Autodesk Inventor part; units mm, degrees
ref_plane "YZ Plane" through (0, 0, 0) normal (1, 0, 0) x (0, 1, 0)
ref_plane "XZ Plane" through (0, 0, 0) normal (0, 1, 0) x (-1, 0, 0)
ref_plane "XY Plane" through (0, 0, 0) normal (0, 0, 1) x (1, 0, 0)
sketch "Sketch1" plane through (0, 0, 0) normal (0, 0, 1) x (1, 0, 0)
  line L0 (0, 0) -> (120.65, 0)
  line L1 (120.65, 0) -> (120.65, 113.9317)
  line L2 (0, 113.9317) -> (0, 0)
  circle A0 centre (11.2141, 60.325) radius 1.9431
  circle A1 centre (60.325, 11.2141) radius 1.9431
  circle A2 centre (109.4359, 60.325) radius 1.9431
  circle A3 centre (60.325, 109.4359) radius 1.9431
  line L3 (60.071, 55.0418) -> (70.739, 55.0418)
  line L4 (70.739, 44.8818) -> (60.071, 44.8818)
  line L5 (60.071, 55.0418) -> (60.071, 44.8818)
  line L6 (70.739, 55.0418) -> (70.739, 44.8818)
  line L7 (60.325, 113.9317) -> (120.65, 113.9317)
  line L8 (60.325, 113.9317) -> (0, 113.9317)
  point P0 (60.325, 60.325)
  dimension "d10" = 3.8862
  dimension "d13" = 360
  dimension "d44" = 4.4958
extrude "Extrusion6" add sketch "Sketch1" along normal blind 25.4
properties part number "speakerback"
Here's how the part is built. I have some questions about the finished solid (model axes, mm). A direction names the side the tool comes from. Coordinates: 2 decimals unless noted, no trailing zeros. Loops run counter-clockwise (first coordinate to the right, second up) from the corner with the lowest first, then second, coordinate; pieces in that order, holes last. Notation, with made-up numbers: M -16,9 L 9,9 A11 cw 9,21 Z; hole C -19.75,1.25 d3. An arc over 180 degrees is marked long. One line per item, written item: value.
1. Please list where these lines run through material, in increasing order: probe 1 along X at (y, z) = (53.5, 15); probe 2 along Y at (x, z) = (64.5, 13.75); probe 3 along X at (y, z) = (10.5, 15).
Geometry says:
probe 1: x = 0 to 60.07, 70.74 to 120.65
probe 2: y = 0 to 44.88, 55.04 to 113.93
probe 3: x = 0 to 58.52, 62.13 to 120.65
2. On a 3-axis mill with a long thin cutter (end or side, diameter ignored), from which of +Z, -Z, +X, -X, +Y, -Y can I reach the whole of each face in a straight line? I mean faces 4 (the flat face through (0, 58, 13)), 5 (the flat face through (65, 55.042, 13)). Say none if no direction works.
Geometry says:
face 4: +Z, -Z, -X, +Y, -Y
face 5: +Z, -Z
3. Imagine slicing it at A-A (x = 65.5). List the corners of the cut face in (y, z) for me, and give its area (3 significant figures).
Geometry says:
outline: M 0,0 L 44.88,0 L 44.88,25.4 L 0,25.4 Z; M 55.04,0 L 113.93,0 L 113.93,25.4 L 55.04,25.4 Z
area: 2,640 mm2
4. Thinking about a two-plate mould opening in Y: for faces 1 (the flat face through (59, 0, 13)), 2 (the flat face through (65, 44.882, 13)), 3 (the flat face through (59, 58, 25.4)), which applies, +Y half, -Y half, draft (parallel to the pull), parting line (faces both ways), or undercut?
Geometry says:
face 1: -Y half
face 2: undercut
face 3: draft
